Geometry: final body of the model. Coordinates: model frame, mm. A direction names the side the tool comes from. Give positions to 0.01 mm unless a question says otherwise; leave off trailing zeros. Write each loop counter-clockwise with the first axis right and the second up, starting at its lowest first coordinate (ties: lowest second). Pieces come first, ordered by that corner, then holes. Notation, with made-up numbers: M 88.5,17.5 L 113.5,17.5 A14 ccw 113.5,34.5 Z; hole C -38.5,65 d6. An arc over 180 degrees is marked long. One line per question, with ' | ' between items.
from build123d import *

# Parameters (mm, degrees)
CHAMFER1_SIZE      = 0.5
CUT_EXTRUDE1_DEPTH = 2.5


with BuildPart() as part:
    # Sketch1 → Revolve1 (revolve)
    with BuildSketch(Plane.XY):
        Polygon((-5, 0), (-5, 3.75), (-4.5, 4.25), (0, 4.25), (0, 2.5), (20, 2.5), (20, 0), align=None)
    revolve(axis=Axis((20, 0, 0), (-1, 0, 0)))

    # Chamfer1
    chamfer1_edges = [part.edges().sort_by_distance(p)[0] for p in [
        (20, -2.5, 0),
    ]]
    chamfer(chamfer1_edges, length=CHAMFER1_SIZE)

    # Sketch2 → Cut-Revolve1 (revolve, cut)
    with BuildSketch(Plane.XY):
        Polygon((-5, 0), (-5, 2), (-2.5, 2), (-1.964101615, 0), align=None)
    revolve(axis=Axis((-1.964101615, 0, 0), (-1, 0, 0)), mode=Mode.SUBTRACT)

    # Sketch3 → Cut-Extrude1 (cut)
    with BuildSketch(Plane(origin=(-5, 0, 0), x_dir=(0, 0, -1), z_dir=(1, 0, 0))):
        Polygon((-2, 1.154700538), (-2, -1.154700538), (0, -2.309401077), (2, -1.154700538), (2, 1.154700538), (0, 2.309401077), align=None)
    extrude(amount=CUT_EXTRUDE1_DEPTH, mode=Mode.SUBTRACT)


solid = part.part
(1) First-contact query: P1, Ø1.5, axis at x = 2, z = 0.5, coming from the +Y side; P2, Ø4, axis at x = 9.5, z = 3.5, coming from the -Y side; P3, Ø2, axis at x = -0.5, z = -2.5, coming from the +Y side. Flat tips, straight axial feed; report the tip coordinate or a pass-through.
Working result:
P1: stops at y = 2.5 | P2: stops at y = -2 | P3: stops at y = 3.98
(2) Draft query along Y for faces 1 (the face through (-4, 0, 2)), 2 (the face through (-5, -2, 2)), 3 (the face through (-3.77, -1.74, -0.99)), 4 (the face through (-2.218, 2.285, -3.584)). Return one class per face: released by +Y, released by -Y, zero draft, split by the parting line, or undercut.
Working result:
face 1: undercut | face 2: zero draft | face 3: undercut | face 4: split by the parting line
(3) Material intervals for L1, parallel to X at y = -0.25, z = -3.5; L2, parallel to Z at x = 4, y = 0, sorted ascending. Write a range as [from, to].
Working result:
L1: x = [-5, 0] | L2: z = [-2.5, 2.5]
(4) Set-up query: faces 5 (the face through (-3.768, -1.724, 1.014)), 6 (the face through (20, 0, 0)), 7 (the face through (0, 2, 2)). Return all of +Z, -Z, +X, -X, +Y, -Y with unobstructed straight access to the full face (end or side cutting, diameter ignored); none if empty.
Working result:
face 5: -X | face 6: +Z, -Z, +X, +Y, -Y | face 7: +X
(5) Cut plane A-A, the plane x = 7.5. Return loops of the section in (y, z).
Working result:
outline: C 0,0 d5
